```python
from build123d import *

# Parameters (mm, degrees)
EXTRUDE_1_DEPTH     = 260
SKETCH_2_R          = 1.5
CUT_EXTRUDE_1_DEPTH = 6
SKETCH_3_R          = 1.5
CUT_EXTRUDE_2_DEPTH = 4
SKETCH_5_R          = 1.5
CUT_EXTRUDE_4_DEPTH = 4


with BuildPart() as part:
    # Эскиз1 → Бобышка-Вытянуть1 (new body)
    with BuildSketch(Plane(origin=(0, 0, 0), x_dir=(0, 0, -1), z_dir=(1, 0, 0))):
        Polygon((0, 0), (-11, 0), (-11, 3), (-5, 3), (-5, 9.5), (-2, 9.5), (-2, 11), (0, 11), align=None)
    extrude(amount=EXTRUDE_1_DEPTH)

    # Эскиз2 → Вырез-Вытянуть1 (cut, through all)
    with BuildSketch(Plane.XY.offset(5)):
        with Locations((256.5, 6.25)):
            Circle(SKETCH_2_R)
    extrude(amount=-CUT_EXTRUDE_1_DEPTH, mode=Mode.SUBTRACT)

    # Эскиз3 → Вырез-Вытянуть2 (cut, through all)
    with BuildSketch(Plane(origin=(0, 3, 0), x_dir=(1, 0, 0), z_dir=(0, 1, 0))):
        with Locations((7.5, -8)):
            Circle(SKETCH_3_R)
        with Locations((18.75, -8)):
            Circle(SKETCH_3_R)
    extrude(amount=-CUT_EXTRUDE_2_DEPTH, mode=Mode.SUBTRACT)

    # Эскиз5 → Вырез-Вытянуть4 (cut, through all)
    with BuildSketch(Plane(origin=(0, 3, 0), x_dir=(1, 0, 0), z_dir=(0, 1, 0))):
        with Locations((65, -8)):
            Circle(SKETCH_5_R)
        with Locations((220, -8)):
            Circle(SKETCH_5_R)
    extrude(amount=-CUT_EXTRUDE_4_DEPTH, mode=Mode.SUBTRACT)


solid = part.part
```
Input: part model. Units: mm. Frame: model coordinates. A direction names the side the tool comes from. Give positions to 0.01 mm unless a question says otherwise; leave off trailing zeros. Order: outer loops, then holes, each group sorted by start corner. A loop starts at its lowest first (then second) coordinate and runs counter-clockwise, first axis right, second up. Notation, with made-up numbers: (42.25, 83) -> (89.25, 83) arc R13 ccw to (89.25, 95) -> close; hole circle Ø1 at (29.5, -1.5). An arc over 180 degrees is marked (long way). Write each question's results on one line, items separated by ' | '. Start each with the question number.
Item 1: Line query: line 1 (X direction, y = 0.65, z = 8); line 2 (Y direction, x = 256.5, z = 3.65); line 3 (Z direction, x = 7.5, y = 1.9). Output: solid intervals per line, ascending.
Item 2: Cut plane A-A on x = 196.5. Return the cut outline in (y, z).
Item 3: Contact query for flat-ended pins moving along their axis: P1, Ø2.5, axis at x = 65, z = 8, coming from the +Y side; P2, Ø3.5, axis at x = 18.75, z = 8, coming from the +Y side; P3, Ø1.5, axis at x = 99, y = 6.5, coming from the +Z side; P4, Ø1.5, axis at x = 188.5, z = 4, coming from the +Y side. Output: stop coordinate, or through.
Item 4: Set-up query: faces 1 (the flat face through (0, 4, 3)), 2 (the flat face through (128, 6, 5)). Return all of +Z, -Z, +X, -X, +Y, -Y with unobstructed straight access to the full face (end or side cutting, diameter ignored); none if empty.
Established:
1) line 1: 0 to 6, 9 to 17.25, 20.25 to 63.5, 66.5 to 218.5, 221.5 to 260 | line 2: 0 to 4.75, 7.75 to 9.5 | line 3: 0 to 6.5, 9.5 to 11
2) outline: (0, 0) -> (11, 0) -> (11, 2) -> (9.5, 2) -> (9.5, 5) -> (3, 5) -> (3, 11) -> (0, 11) -> close
3) P1: through | P2: y = 3 | P3: z = 5 | P4: y = 9.5
4) face 1: +Z, -Z, -X, +Y, -Y | face 2: +Z, +X, -X, +Y
